Verification items for the finished model (mm, model axes). A direction names the side the tool comes from. Give positions to 0.01 mm unless a question says otherwise; leave off trailing zeros. Order: outer loops, then holes, each group sorted by start corner. A loop starts at its lowest first (then second) coordinate and runs counter-clockwise, first axis right, second up. Notation, with made-up numbers: (-29, -38) -> (5, -38) arc R18 cw to (5, -10) -> close; hole circle Ø9 at (85.5, 45). An arc over 180 degrees is marked (long way). Write each question's results on one line, items separated by ' | '. Start each with the question number.
1. Depth check by flat-ended pin: pin 1 Ø25 at (x, z) = (89.5, -20) entering from +Y; pin 2 Ø8 at (y, z) = (22, -33) entering from +X. Enter the tip coordinate at first touch or a pass-through.
2. Cross-section at A-A, the plane x = 25. Enter the section's corners in (y, z), then the cut area to 3 significant figures.
3. Material ranges on L1, parallel to X at y = 7.5, z = -25; L2, parallel to X at y = 5.75, z = -12.5; L3, parallel to Y at x = 126.5, z = -46.5, recorded low to high. Write a range as from..to.
4. Cross-section at B-B, the plane z = -25. Enter the section's corners in (x, y), then the cut area to 3 significant figures.
5. Cross-section at D-D, the plane y = 21.25. Enter the section's corners in (x, z), then the cut area to 3 significant figures.
6. Mould release check, pull along Z, two halves, no side actions. Record for faces 3 (the face through (23.048, 13.212, -37.066)), 4 (the face through (99, 10, -50)), 5 (the face through (200, 8, -25)): +Z half, -Z half, draft (parallel to the pull), parting line (faces both ways), or undercut.
7. Set-up check for faces 1 (the face through (124, 16.85, -25)), 2 (the face through (0, 13, -25)): record each of +Z, -Z, +X, -X, +Y, -Y from which the full face is reachable in a straight line by a thin tool's end or side.
8. Cross-section at C-C, the plane x = 170. Enter the section's corners in (y, z).
from build123d import *

# Parameters (mm, degrees)
SKETCH1_W           = 50
SKETCH1_H           = 50
BOSS_EXTRUDE1_DEPTH = 26.8
SKETCH1_3_W         = 150
SKETCH1_3_H         = 50
BOSS_EXTRUDE2_DEPTH = 16.85
SKETCH2_R           = 2
SKETCH2_R_2         = 3
CUT_EXTRUDE1_DEPTH  = 208.889970898


with BuildPart() as part:
    # Sketch1 → Boss-Extrude1 (new body)
    with BuildSketch(Plane(origin=(0, 0, 0), x_dir=(1, 0, 0), z_dir=(0, 1, 0))):
        with Locations((25, 25)):
            Rectangle(SKETCH1_W, SKETCH1_H)
    extrude(amount=BOSS_EXTRUDE1_DEPTH)

    # Sketch1_3 → Boss-Extrude2 (add)
    with BuildSketch(Plane(origin=(0, 0, 0), x_dir=(1, 0, 0), z_dir=(0, 1, 0))):
        with Locations((125, 25)):
            Rectangle(SKETCH1_3_W, SKETCH1_3_H)
    extrude(amount=BOSS_EXTRUDE2_DEPTH)

    # Sketch2 → Cut-Extrude1 (cut, through all)
    with BuildSketch(Plane.XZ):
        with Locations(Location((25, -37.5, 0), (0, 0, 270))):
            Circle(SKETCH2_R)
        with Locations(Location((25, -12.5, 0), (0, 0, 270))):
            Circle(SKETCH2_R)
        with Locations(Location((170, -25, 0), (0, 0, 270))):
            Circle(SKETCH2_R_2)
    extrude(amount=-CUT_EXTRUDE1_DEPTH, mode=Mode.SUBTRACT)


solid = part.part
Results below:
1) pin 1: stops at y = 16.85 | pin 2: stops at x = 50
2) outline: (0, -50) -> (26.8, -50) -> (26.8, -39.5) -> (0, -39.5) -> close; (0, -35.5) -> (26.8, -35.5) -> (26.8, -14.5) -> (0, -14.5) -> close; (0, -10.5) -> (26.8, -10.5) -> (26.8, 0) -> (0, 0) -> close | area: 1,130 mm²
3) L1: x = 0..167, 173..200 | L2: x = 0..23, 27..200 | L3: y = 0..16.85
4) outline: (0, 0) -> (167, 0) -> (167, 16.85) -> (50, 16.85) -> (50, 26.8) -> (0, 26.8) -> close; (173, 0) -> (200, 0) -> (200, 16.85) -> (173, 16.85) -> close | area: 3,770 mm²
5) outline: (0, -50) -> (50, -50) -> (50, 0) -> (0, 0) -> close; hole circle Ø4 at (25, -37.5); hole circle Ø4 at (25, -12.5) | area: 2,470 mm²
6) face 3: undercut | face 4: -Z half | face 5: draft
7) face 1: +Z, -Z, +X, +Y | face 2: +Z, -Z, -X, +Y, -Y
8) outline: (0, -50) -> (16.85, -50) -> (16.85, -28) -> (0, -28) -> close; (0, -22) -> (16.85, -22) -> (16.85, 0) -> (0, 0) -> close
